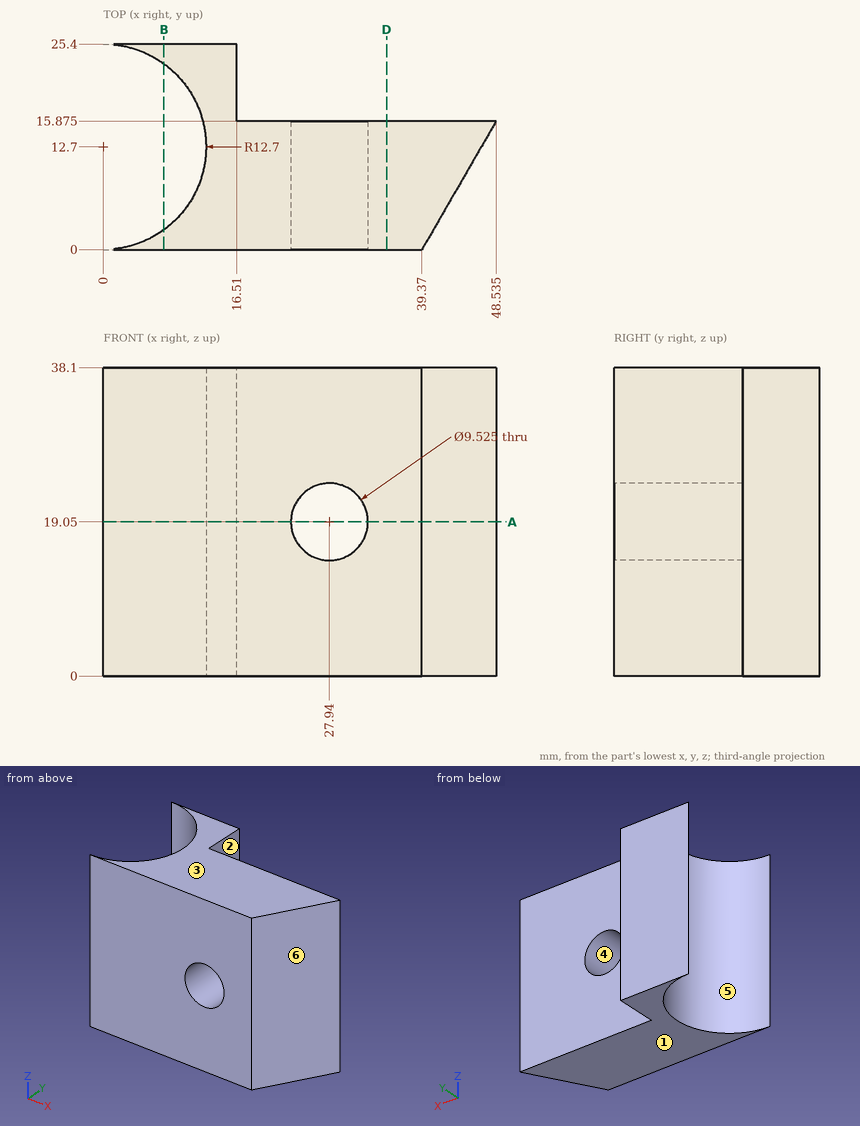
Verification items for this drawing (mm, ordinates from the low corner). A direction names the side the tool comes from. Give positions to 0.01 mm unless a question says otherwise; leave off trailing zeros. Loops run counter-clockwise (first coordinate to the right, second up) from the corner with the lowest first, then second, coordinate; pieces in that order, holes last. Notation, with made-up numbers: M -29,25 L -14,25 A15 ccw -14,32 Z; hole C -20,61 d3. An arc over 180 degrees is marked long. Answer as a JSON object with one key per item and string values. Group by question number.
Item 1: Sectioned sample at D-D on x = 35. Record the boundary of the cut face in (y, z) (1 decimal).
Item 2: Mould release check, pull along X, two halves, no side actions. Record for the marked faces 3, 4, 5 and 6: pulls with the +X half, pulls with the -X half, needs draft (parallel to the pull), parting line crosses it, or undercut.
Item 3: Material ranges on L1, parallel to Y at x = 29.5, z = 11.5 (1 decimal); L2, parallel to Z at x = 29.5, y = 4; L3, parallel to X at y = 5, z = 19.05 (1 decimal), recorded low to high.
Item 4: Access from +Z, -Z, +X, -X, +Y, -Y to the whole of each face (thin tool, end or side, straight path). Record for the marked faces 1 and 2.
Item 5: Sectioned sample at A-A on z = 19.05. Record the boundary of the cut face in (x, y) (1 decimal).
Item 6: Sectioned sample at B-B on x = 7.5. Record the boundary of the cut face in (y, z).
Item 7: Gauge pin test, flat ends, axial feed: pin 1 (5 mm diameter, centred on y = 21.5, z = 23, fed in from +X); pin 2 (1 mm diameter, centred on y = 3, z = 29, fed in from -X) (1 decimal); pin 3 (16 mm diameter, centred on x = 36.5, z = 25.5, fed in from +Y) (3 decimals). Record the tip position at first contact, or that the pin passes through.
Findings below:
{
 "1": {"outline": "M 0,0 L 15.9,0 L 15.9,38.1 L 0,38.1 Z"},
 "2": {"face 3": "needs draft", "face 4": "undercut", "face 5": "pulls with the -X half", "face 6": "pulls with the +X half"},
 "3": {"L1": "0 to 15.9", "L2": "0 to 14.55, 23.55 to 38.1", "L3": "10.1 to 23.2, 32.7 to 42.3"},
 "4": {"face 1": "-Z, +X, -X, +Y, -Y", "face 2": "+Z, -Z, +X, +Y"},
 "5": {"outline": "M 0,0 L 23.2,0 L 23.2,15.9 L 16.5,15.9 L 16.5,25.4 L 0,25.4 A12.7 cw Z; M 32.7,0 L 39.4,0 L 48.5,15.9 L 32.7,15.9 Z"},
 "6": {"outline": "M 0,0 L 2.45,0 L 2.45,38.1 L 0,38.1 Z; M 22.95,0 L 25.4,0 L 25.4,38.1 L 22.95,38.1 Z"},
 "7": {"pin 1": "x = 16.51", "pin 2": "x = 7.6", "pin 3": "y = 15.875"}
}
